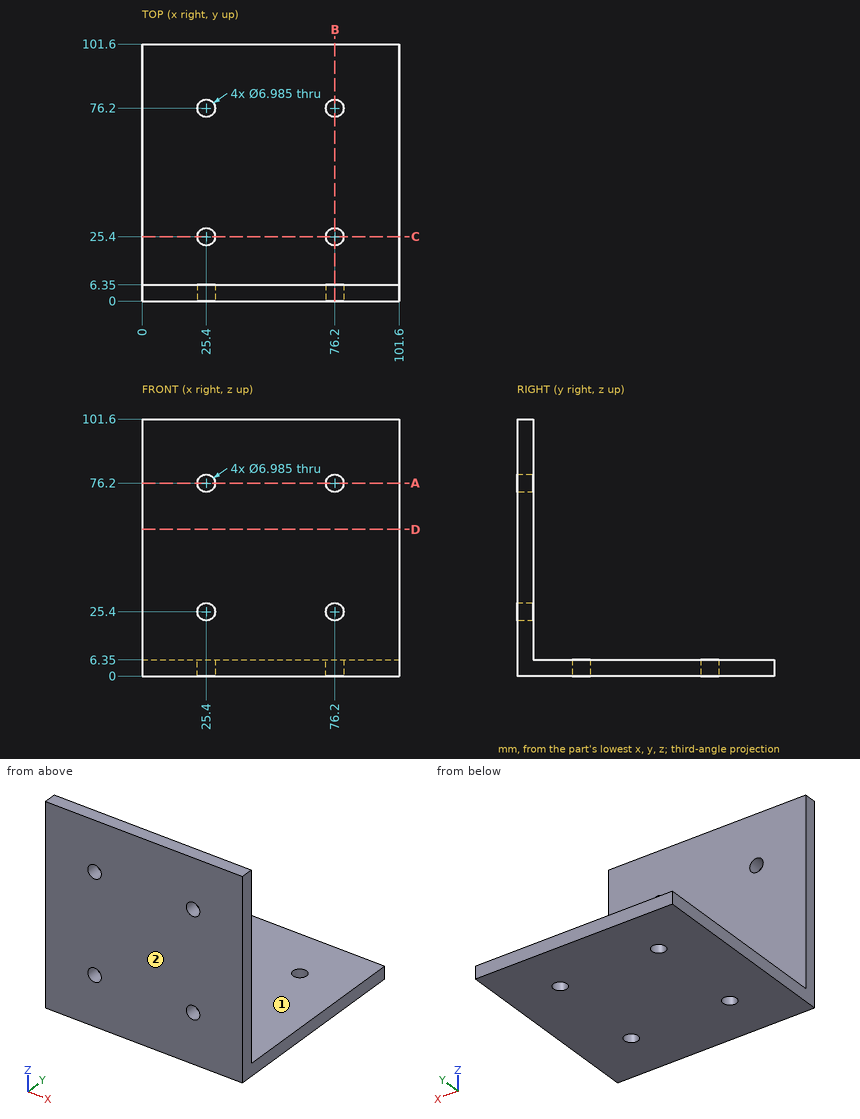
Here's the drawing with two shaded views (mm, measured from the low corner). I have some questions. A direction names the side the tool comes from. Give positions to 0.01 mm unless a question says otherwise; leave off trailing zeros. Loops run counter-clockwise (first coordinate to the right, second up) from the corner with the lowest first, then second, coordinate; pieces in that order, holes last. Notation, with made-up numbers: (68.5, 54) - (116.5, 54) arc R12 ccw to (116.5, 61) - close; hole circle Ø9 at (21, 39). An arc over 180 degrees is marked (long way). Return JSON: item names as keys, results as strings.
1. I want a section at D-D on z = 58. Please give me the cut outline in (x, y), and give its area (3 significant figures).
Output values:
{"outline": "(0, 0) - (101.6, 0) - (101.6, 6.35) - (0, 6.35) - close", "area": "645 mm²"}
2. I'm going to push flat-ended pins straight in: pin 1 Ø2 at (x, z) = (25, 74.5) entering from +Y; pin 2 Ø11 at (x, y) = (76.2, 25.4) entering from +Z; pin 3 Ø6 at (x, z) = (30, 14.5) entering from +Y. Where does each tip first touch, or does it pass through?
Output values:
{"pin 1": "passes through", "pin 2": "stops at z = 6.35", "pin 3": "stops at y = 6.35"}
3. For the marked faces 1 and 2, which set-ups out of +Z, -Z, +X, -X, +Y, -Y let a thin tool reach every point of the face, with its end or its side?
Output values:
{"face 1": "+Z, +X, -X, +Y", "face 2": "+Z, -Z, +X, -X, -Y"}
4. I want a section at A-A on z = 76.2. Please give me the cut outline in (x, y), and give its area (3 significant figures).
Output values:
{"outline": "(0, 0) - (21.91, 0) - (21.91, 6.35) - (0, 6.35) - close; (28.89, 0) - (72.71, 0) - (72.71, 6.35) - (28.89, 6.35) - close; (79.69, 0) - (101.6, 0) - (101.6, 6.35) - (79.69, 6.35) - close", "area": "556 mm²"}
5. I want a section at B-B on x = 76.2. Please give me the cut outline in (y, z), and give its area (3 significant figures).
Output values:
{"outline": "(0, 0) - (21.91, 0) - (21.91, 6.35) - (6.35, 6.35) - (6.35, 21.91) - (0, 21.91) - close; (0, 28.89) - (6.35, 28.89) - (6.35, 72.71) - (0, 72.71) - close; (0, 79.69) - (6.35, 79.69) - (6.35, 101.6) - (0, 101.6) - close; (28.89, 0) - (72.71, 0) - (72.71, 6.35) - (28.89, 6.35) - close; (79.69, 0) - (101.6, 0) - (101.6, 6.35) - (79.69, 6.35) - close", "area": "1,070 mm²"}
6. If I drill on line 1 (X direction, y = 3.75, z = 76.2), over which ranges is the centre line in solid material (lowest first)?
Output values:
{"line 1": "x = 0 to 21.91, 28.89 to 72.71, 79.69 to 101.6"}
